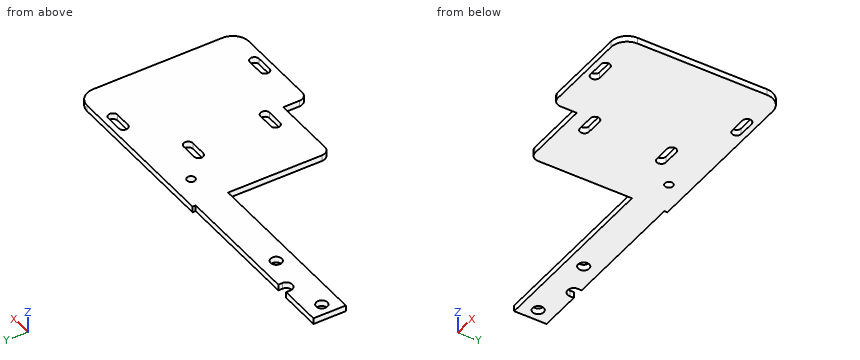
```python
from build123d import *

# Parameters (mm, degrees)
F0_R     = 4.365625
F0_R_2   = 3.175
F1_DEPTH = 4.7625


with BuildPart() as f1:
    # F0 (on Top) → F1 (new body)
    with BuildSketch(Plane.XY):
        with BuildLine():
            Line((128.5875, 0), (0, 0))
            Line((0, 0), (0, -2.3876))
            Line((0, -2.3876), (-100.81895, -2.3876))
            Line((-100.81895, -2.3876), (-100.81895, -5.5626))
            ThreePointArc((-100.81895, -5.5626), (-105.58145, -10.3251), (-110.34395, -5.5626))
            Line((-110.34395, -5.5626), (-110.34395, -2.3876))
            Line((-110.34395, -2.3876), (-143.68145, -2.3876))
            Line((-143.68145, -2.3876), (-143.68145, -27.7876))
            Line((-143.68145, -27.7876), (0, -27.7876))
            Line((0, -27.7876), (0, -101.6))
            ThreePointArc((0, -101.6), (1.859872, -106.090128), (6.35, -107.95))
            Line((6.35, -107.95), (57.15, -107.95))
            Line((57.15, -107.95), (57.15, -120.65))
            ThreePointArc((57.15, -120.65), (59.009872, -125.140128), (63.5, -127))
            Line((63.5, -127), (128.5875, -127))
            ThreePointArc((128.5875, -127), (137.567756, -123.280256), (141.2875, -114.3))
            Line((141.2875, -114.3), (141.2875, -12.7))
            ThreePointArc((141.2875, -12.7), (137.567756, -3.719744), (128.5875, 0))
        make_face()
        with BuildLine():
            ThreePointArc((109.5375, -115.490625), (113.109375, -119.0625), (109.5375, -122.634375))
            Line((109.5375, -122.634375), (96.8375, -122.634375))
            ThreePointArc((96.8375, -122.634375), (93.265625, -119.0625), (96.8375, -115.490625))
            Line((96.8375, -115.490625), (109.5375, -115.490625))
        make_face(mode=Mode.SUBTRACT)
        with BuildLine():
            ThreePointArc((57.15, -90.090625), (60.721875, -93.6625), (57.15, -97.234375))
            Line((57.15, -97.234375), (44.45, -97.234375))
            ThreePointArc((44.45, -97.234375), (40.878125, -93.6625), (44.45, -90.090625))
            Line((44.45, -90.090625), (57.15, -90.090625))
        make_face(mode=Mode.SUBTRACT)
        with Locations((-134.15645, -15.0876)):
            Circle(F0_R, mode=Mode.SUBTRACT)
        with Locations((-78.59395, -15.0876)):
            Circle(F0_R, mode=Mode.SUBTRACT)
        with BuildLine():
            ThreePointArc((57.15, -29.765625), (60.721875, -33.3375), (57.15, -36.909375))
            Line((57.15, -36.909375), (44.45, -36.909375))
            ThreePointArc((44.45, -36.909375), (40.878125, -33.3375), (44.45, -29.765625))
            Line((44.45, -29.765625), (57.15, -29.765625))
        make_face(mode=Mode.SUBTRACT)
        with Locations((25.4, -15.0876)):
            Circle(F0_R_2, mode=Mode.SUBTRACT)
        with BuildLine():
            ThreePointArc((109.5375, -4.365625), (113.109375, -7.9375), (109.5375, -11.509375))
            Line((109.5375, -11.509375), (96.8375, -11.509375))
            ThreePointArc((96.8375, -11.509375), (93.265625, -7.9375), (96.8375, -4.365625))
            Line((96.8375, -4.365625), (109.5375, -4.365625))
        make_face(mode=Mode.SUBTRACT)
    extrude(amount=-F1_DEPTH)


solid = f1.part
```
The model under review builds one solid part; all positions refer to its coordinate system, in mm. Give positions to 0.01 mm unless a question says otherwise; leave off trailing zeros. Write each loop counter-clockwise with the first axis right and the second up, starting at its lowest first coordinate (ties: lowest second). Pieces come first, ordered by that corner, then holes. Notation, with made-up numbers: (35, 30.25) -> (77, 30.25) arc R16 cw to (77, 43.25) -> close; hole circle Ø2 at (81, 14.5). An arc over 180 degrees is marked (long way). Answer in a Markdown table with one row per item.
1) Add section D-D on z = -0.75. Count the separate pieces of the cut face and the enclosed holes in it, plus the area to 3 significant figures.
Worked answers:
| item | result |
|---|---|
| separate pieces | 1 |
| enclosed holes | 7 |
| area | 19,700 mm² |
2) Add section B-B on y = -56.5. State the section outline as (x, z) points.
Worked answers:
| item | result |
|---|---|
| outline | (0, -4.76) -> (141.29, -4.76) -> (141.29, 0) -> (0, 0) -> close |
3) Clearance check with flat-ended pins moving along their axes: P1, Ø1.4, axis at x = 20, z = -1.5, coming from the -Y side; P2, Ø2, axis at y = -45, z = -3, coming from the -X side; P3, Ø2, axis at y = -112.5, z = -3, coming from the -X side. State where each tip first meets the part, or that it passes through.
Worked answers:
| item | result |
|---|---|
| P1 | y = -107.95 |
| P2 | x = 0 |
| P3 | x = 57.15 |
4) Add section C-C on x = -53. State the section outline as (y, z) points.
Worked answers:
| item | result |
|---|---|
| outline | (-27.79, -4.76) -> (-2.39, -4.76) -> (-2.39, 0) -> (-27.79, 0) -> close |
5) For L1, parallel to Y at x = 102.5, z = -4; L2, parallel to Y at x = 56, z = -1.05; L3, parallel to Y at x = 25.4, z = -3.2, list the stretches that pass through material, from the lowest coordinate up. Write a range as [from, to].
Worked answers:
| item | result |
|---|---|
| L1 | [-127, -122.63], [-115.49, -11.51], [-4.37, 0] |
| L2 | [-107.95, -97.23], [-90.09, -36.91], [-29.77, 0] |
| L3 | [-107.95, -18.26], [-11.91, 0] |
6) Add section A-A on x = 25.4. State the section outline as (y, z) points.
Worked answers:
| item | result |
|---|---|
| outline | (-107.95, -4.76) -> (-18.26, -4.76) -> (-18.26, 0) -> (-107.95, 0) -> close; (-11.91, -4.76) -> (0, -4.76) -> (0, 0) -> (-11.91, 0) -> close |
